Autodesk Inventor part; units mm, degrees
ref_plane "YZ Plane" through (0, 0, 0) normal (1, 0, 0) x (0, 1, 0)
ref_plane "XZ Plane" through (0, 0, 0) normal (0, 1, 0) x (-1, 0, 0)
ref_plane "XY Plane" through (0, 0, 0) normal (0, 0, 1) x (1, 0, 0)
sketch "Sketch1" plane through (0, 0, 0) normal (1, 0, 0) x (0, 1, 0)
  circle A0 centre (0, 0) radius 5.25
  line L0 (0, 0) -> (16.2396, 0) construction
  line L1 (5.4642, 5.1373) -> (101.0943, 5.1373)
  line L2 (5.4642, -5.1373) -> (101.0943, -5.1373)
  circle A1 centre (123, 0) radius 22.5
  circle A2 centre (123, 0) radius 17.75
  circle A3 centre (0, 0) radius 7.5
  dimension "d20" = 15
  dimension "d0" = 10.5
  dimension "d14" = 45
  dimension "d16" = 35.5
  dimension "d17" = 123
extrude "Extrusion1" add sketch "Sketch1" along normal mid plane 25 contours A3 | A1
extrude "Extrusion2" add sketch "Sketch1" along normal mid plane 10 contours L1 A1 L2 A3
sketch "Sketch2" plane through (0, 0, 0) normal (0, 0, 1) x (1, 0, 0)
  line L0 (-12.5, 145.5) -> (12.5, 145.5)
  line L1 (0, 113.4787) -> (0, 177.5213) construction
  line L2 (-17.5, 144.5) -> (17.5, 144.5)
  line L3 (17.5, 144.5) -> (17.5, 146.5)
  line L4 (17.5, 146.5) -> (-17.5, 146.5)
  line L5 (-17.5, 146.5) -> (-17.5, 144.5)
  point P0 (0, 0)
  point P1 (0, 145.5)
  point P2 (0, 146.5)
  dimension "d21" = 1
  dimension "d22" = 2
  dimension "d23" = 35
extrude "Extrusion3" add sketch "Sketch2" along normal mid plane 30
sketch "Sketch3" plane through (-17.5, 146.5, 15) normal (0, 1, 0) x (1, 0, 0)
  circle A0 centre (22.5, 15) radius 2.5
  circle A1 centre (12.5, 15) radius 2.5
  line L0 (17.5, -7.5) -> (17.5, 37.5) construction
  line L1 (5, 37.5) -> (30, 37.5)
  point P0 (17.5, 15)
  dimension "d26" = 5
  dimension "d27" = 5
  dimension "d28" = 5
  dimension "d29" = 5
extrude "Extrusion4" add sketch "Sketch3" along normal blind 64
properties part number "guide"
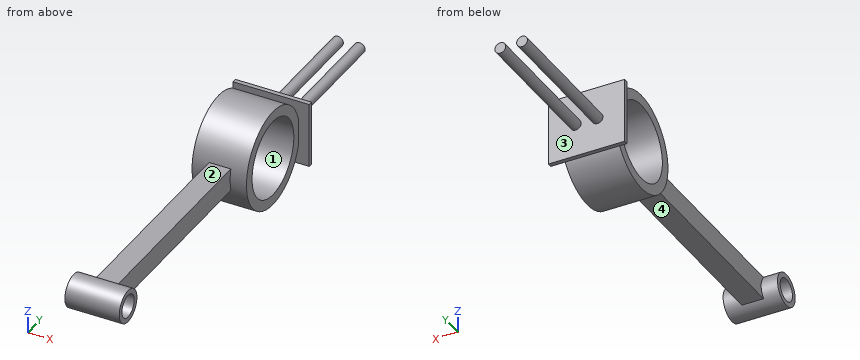
Here's how the part is built. I have some questions about the finished solid (model axes, mm). Face numbers are marked on the shaded views. A direction names the side the tool comes from. Coordinates: 2 decimals unless noted, no trailing zeros. Write each loop counter-clockwise with the first axis right and the second up, starting at its lowest first coordinate (ties: lowest second). Pieces come first, ordered by that corner, then holes.
Item 1: I want a section at B-B on z = 0. Count the separate pieces of the cut face and the enclosed holes in it, and give its area (4 significant figures).
Item 2: I want a section at C-C on y = 123. Write out the boundary of the cut face in (x, z).
Item 3: I want a section at D-D on y = 57. Write out the boundary of the cut face in (x, z).
Item 4: I want a section at A-A on y = 0. Write out the boundary of the cut face in (x, z).
Item 5: If I drill on line 1 (Z direction, x = 1.75, y = 0); line 2 (Z direction, x = -7, y = 123); line 3 (Y direction, x = 5, z = 14), over which ranges is the centre line in solid material (lowest first)?
Item 6: On a 3-axis mill with a long thin cutter (end or side, diameter ignored), from which of +Z, -Z, +X, -X, +Y, -Y can I reach the whole of each face in a straight line? I mean the marked faces 1 and 2. Say none if no direction works.
Item 7: Will these pins go through, and if not, where does the flat tip stop? pin 1 (4.5 mm diameter, centred on y = -3.5, z = 1, fed in from -X); pin 2 (6.5 mm diameter, centred on y = 0, z = 0, fed in from +X); pin 3 (5 mm diameter, centred on y = 59.5, z = 0.5, fed in from +X); pin 4 (8 mm diameter, centred on y = 34, z = -1, fed in from -X).
Item 8: If we mould it in two halves opening along Y, with no side actions, what happens to the marked faces 3 and 4? For each: +Y half, -Y half, draft (parallel to the pull), parting line (faces both ways), or undercut.
Findings below:
1. separate pieces: 3
1. enclosed holes: 0
1. area: 1,965 mm2
2. outline: (-12.5, -22.5) - (12.5, -22.5) - (12.5, -17.75) - (-12.5, -17.75) - close; (-12.5, 17.75) - (12.5, 17.75) - (12.5, 22.5) - (-12.5, 22.5) - close
3. outline: (-5, -5.14) - (5, -5.14) - (5, 5.14) - (-5, 5.14) - close
4. outline: (-12.5, -7.5) - (12.5, -7.5) - (12.5, -5.25) - (-12.5, -5.25) - close; (-12.5, 5.25) - (12.5, 5.25) - (12.5, 7.5) - (-12.5, 7.5) - close
5. line 1: z = -7.5 to -5.25, 5.25 to 7.5
5. line 2: z = -22.5 to -17.75, 17.75 to 22.5
5. line 3: y = 105.39 to 112.09, 133.91 to 140.61, 144.5 to 146.5
6. face 1: +X, -X
6. face 2: +Z, +X, -X
7. pin 1: stops at x = -12.5
7. pin 2: passes through
7. pin 3: stops at x = 5
7. pin 4: stops at x = -5
8. face 3: +Y half
8. face 4: undercut
